```python
from build123d import *

# Parameters (mm, degrees)
ESQUISSE1_W                = 20
ESQUISSE1_H                = 600
BOSS_EXTRU_1_DEPTH         = 11
ENL_V_MAT_EXTRU_1_DEPTH    = 601.184138411
ENL_V_MAT_EXTRU_2_DEPTH    = 601.184138411
ENL_V_MAT_EXTRU_3_DEPTH    = 601.184138411
ENL_V_MAT_EXTRU_4_DEPTH    = 601.184138411
PER_AGE1_D                 = 4.917
PER_AGE2_D                 = 4.917
CHANFREIN1_SIZE            = 0.5415
CHANFREIN2_SIZE            = 0.3
R_P_TITION_LIN_AIRE1_COUNT = 9
R_P_TITION_LIN_AIRE1_PITCH = 60


with BuildPart() as part:
    # Esquisse1 → Boss.-Extru.1 (new body)
    with BuildSketch(Plane.XZ):
        with Locations((0, -50)):
            Rectangle(ESQUISSE1_W, ESQUISSE1_H)
    extrude(amount=-BOSS_EXTRU_1_DEPTH)

    # Esquisse2 → Enlèv. mat.-Extru.1 (cut, through all)
    with BuildSketch(Plane(origin=(0, 0, -350), x_dir=(-1, 0, 0), z_dir=(0, 0, -1))):
        with BuildLine():
            Line((10, 7.9), (10, 10.22385))
            Line((10, 10.22385), (9.440021531, 9.900556887))
            ThreePointArc((9.440021531, 9.900556887), (9.015681976, 9.557293765), (8.71772889, 9.1))
            Line((8.71772889, 9.1), (7.5, 9.1))
            Line((7.5, 9.1), (7.5, 7.9))
            Line((7.5, 7.9), (10, 7.9))
        make_face()
    extrude(amount=-ENL_V_MAT_EXTRU_1_DEPTH, mode=Mode.SUBTRACT)

    # Esquisse3 → Enlèv. mat.-Extru.2 (cut, through all)
    with BuildSketch(Plane(origin=(0, 0, -350), x_dir=(-1, 0, 0), z_dir=(0, 0, -1))):
        with BuildLine():
            Line((9.440021531, 7.099443113), (10, 6.77615))
            Line((10, 6.77615), (10, 7.9))
            Line((10, 7.9), (8.71772889, 7.9))
            ThreePointArc((8.71772889, 7.9), (9.015681976, 7.442706235), (9.440021531, 7.099443113))
        make_face()
    extrude(amount=-ENL_V_MAT_EXTRU_2_DEPTH, mode=Mode.SUBTRACT)

    # Esquisse4 → Enlèv. mat.-Extru.3 (cut, through all)
    with BuildSketch(Plane(origin=(0, 0, -350), x_dir=(-1, 0, 0), z_dir=(0, 0, -1))):
        with BuildLine():
            Line((-10, 9.1), (-10, 6.77615))
            Line((-10, 6.77615), (-9.440021531, 7.099443113))
            ThreePointArc((-9.440021531, 7.099443113), (-9.015681976, 7.442706235), (-8.71772889, 7.9))
            Line((-8.71772889, 7.9), (-7.5, 7.9))
            Line((-7.5, 7.9), (-7.5, 9.1))
            Line((-7.5, 9.1), (-10, 9.1))
        make_face()
    extrude(amount=-ENL_V_MAT_EXTRU_3_DEPTH, mode=Mode.SUBTRACT)

    # Esquisse5 → Enlèv. mat.-Extru.4 (cut, through all)
    with BuildSketch(Plane(origin=(0, 0, -350), x_dir=(-1, 0, 0), z_dir=(0, 0, -1))):
        with BuildLine():
            Line((-9.440021531, 9.900556887), (-10, 10.22385))
            Line((-10, 10.22385), (-10, 9.1))
            Line((-10, 9.1), (-8.71772889, 9.1))
            ThreePointArc((-8.71772889, 9.1), (-9.015681976, 9.557293765), (-9.440021531, 9.900556887))
        make_face()
    extrude(amount=-ENL_V_MAT_EXTRU_4_DEPTH, mode=Mode.SUBTRACT)

    # Perçage1 (through all)
    with Locations(Plane(origin=(0, 11, 0), x_dir=(1, 0, 0), z_dir=(0, 1, 0))):
        with Locations((0, -180), (0, -120), (0, 60), (0, 180)):
            Hole(PER_AGE1_D / 2)

    # Perçage2 (through all)
    with Locations(Plane(origin=(0, 0, 0), x_dir=(-1, 0, 0), z_dir=(0, -1, 0))):
        with Locations((0, -240), (0, -60), (0, 0), (0, 120), (0, 240)):
            per_age2 = Hole(PER_AGE2_D / 2)

    # Chanfrein1
    chanfrein1_edges = [part.edges().sort_by_distance(p)[0] for p in [
        (2.4585, 11, 180),
        (2.4585, 0, 180),
        (-2.4585, 0, -240),
        (-2.4585, 11, -240),
        (-2.4585, 0, -120),
        (-2.4585, 11, -120),
        (-2.4585, 0, 0),
        (-2.4585, 11, 0),
        (-2.4585, 0, 60),
        (-2.4585, 11, 60),
        (-2.4585, 0, 240),
        (-2.4585, 11, 240),
        (10, 0, -50),
        (-10, 0, -50),
        (2.4585, 11, -180),
        (2.4585, 0, -180),
        (2.4585, 11, -60),
        (2.4585, 0, -60),
        (2.4585, 11, 120),
        (2.4585, 0, 120),
    ]]
    chamfer(chanfrein1_edges, length=CHANFREIN1_SIZE)

    # Chanfrein2
    chanfrein2_edges = [part.edges().sort_by_distance(p)[0] for p in [
        (10, 11, -50),
        (-10, 11, -50),
    ]]
    chamfer(chanfrein2_edges, length=CHANFREIN2_SIZE)

    # Répétition linéaire1: Perçage2 ×9
    with Locations(*[(0, 0, -i * R_P_TITION_LIN_AIRE1_PITCH) for i in range(1, R_P_TITION_LIN_AIRE1_COUNT)]):
        add(per_age2, mode=Mode.SUBTRACT)


solid = part.part
```
Here's how the part is built. I have some questions about the finished solid (model axes, mm). Give positions to 0.01 mm unless a question says otherwise; leave off trailing zeros.
(1) If I drill on L1, parallel to Y at x = 8.75, z = -304; L2, parallel to X at y = 4, z = 180; L3, parallel to X at y = 8, z = -60, over which ranges is the centre line in solid material (lowest first)?
Output values:
L1: y = 0 to 7.83, 9.17 to 11
L2: x = -10 to -2.46, 2.46 to 10
L3: x = -7.5 to -2.46, 2.46 to 7.5
(2) Imagine slicing it at A-A, the plane y = 3. Count the separate pieces of the cut face and the enclosed holes in it, and give its area (3 significant figures).
Output values:
separate pieces: 1
enclosed holes: 10
area: 11,800 mm2
(3) Will these pins go through, and if not, where does the flat tip stop? pin 1 (4 mm diameter, centred on x = 0, z = 60, fed in from -Y); pin 2 (0.6 mm diameter, centred on y = 8, z = -198, fed in from -X).
Output values:
pin 1: passes through
pin 2: stops at x = -8.82
